```python
from build123d import *

# Parameters (mm, degrees)
EXTRUSION1_REACH = 19.5
ESQUISSE2_R      = 2


with BuildPart() as part:
    # Esquisse1 → Révolution1 (revolve)
    with BuildSketch(Plane.XY):
        Polygon((-17.5, 5), (-4, 5), (-4, 3), (-11, 3), (-11, -21), (-17.5, -21), align=None)
    revolve(axis=Axis((0, 0, 0), (0, -1, 0)))

    # Esquisse2 → Extrusion1 (cut, up to next)
    with BuildSketch(Plane(origin=(0, 0, 0), x_dir=(0, 0, -1), z_dir=(1, 0, 0)), mode=Mode.PRIVATE) as extrusion1_sk1:
        with Locations((0, -13.5)):
            Circle(ESQUISSE2_R)
    extrusion1_tool1 = extrude(extrusion1_sk1.sketch, amount=-EXTRUSION1_REACH, mode=Mode.PRIVATE) & part.part
    add(extrusion1_tool1.solids().sort_by_distance((0, -13.5, 0))[0], mode=Mode.SUBTRACT)


solid = part.part
```
Could you check a few things on this model? Use its own coordinates, in mm. A direction names the side the tool comes from. Round coordinates to 2 decimals unless told otherwise and drop trailing zeros. Write each loop counter-clockwise with the first axis right and the second up, starting at its lowest first coordinate (ties: lowest second). Pieces come first, ordered by that corner, then holes. Notation, with made-up numbers: M 55.5,11.5 L 78.5,11.5 A22 ccw 78.5,36.5 Z; hole C 56,46 d5. An arc over 180 degrees is marked long. Write each question's results on one line, items separated by ' | '. Start each with the question number.
1. Imagine slicing it at B-B on x = 0. List the corners of the cut face in (y, z) for me, and give its area (3 significant figures).
2. Imagine slicing it at D-D on x = 9.5. List the corners of the cut face in (y, z) for me, and give its area (3 significant figures).
3. I'm going to push flat-ended pins straight in: pin 1 Ø5 at (y, z) = (-17.5, 13.5) entering from -X; pin 2 Ø10 at (x, y) = (-6, -14.5) entering from -Z; pin 3 Ø1 at (y, z) = (-0.5, -2.5) entering from +X. Where does each tip first touch, or does it pass through?
4. I need wall thicknesses on L1, parallel to X at y = -5, z = 0; L2, parallel to X at y = 3.9, z = 0. Which ranges of each line are inside material? Lowest first, please. Write a range as from..to.
5. On a 3-axis mill with a long thin cutter (end or side, diameter ignored), from which of +Z, -Z, +X, -X, +Y, -Y can I reach the whole of each face in a straight line? I mean faces 5 (the face through (2.38, -9.17, 10.74)), 6 (the face through (13.887, -7.818, 10.648)). Say none if no direction works.
6. Imagine slicing it at C-C on y = -1.25. List the corners of the cut face in (x, z) for me, and give its area (3 significant figures).
7. Imagine slicing it at A-A on z = 0. List the corners of the cut face in (x, y) for me.
8. Thinking about a two-plate mould opening in Y: for faces 1 (the face through (0.867, 3.986, 3.905)), 2 (the face through (-4, 5, 4)), 3 (the face through (-8, -21, 8)), 4 (the face through (-14.111, -11.517, 0.26)), which applies, +Y half, -Y half, draft (parallel to the pull), parting line (faces both ways), or undercut?
Result sheet:
1) outline: M -21,-17.5 L 5,-17.5 L 5,-4 L 3,-4 L 3,-11 L -21,-11 Z; M -21,11 L 3,11 L 3,4 L 5,4 L 5,17.5 L -21,17.5 Z | area: 366 mm^2
2) outline: M -21,-14.7 L 5,-14.7 L 5,14.7 L -21,14.7 L -21,5.55 L 3,5.55 L 3,-5.55 L -21,-5.55 Z | area: 498 mm^2
3) pin 1: stops at x = -13.61 | pin 2: stops at z = -17.47 | pin 3: stops at x = 17.39
4) L1: x = -17.5..-11, 11..17.5 | L2: x = -17.5..-4, 4..17.5
5) face 5: -Y | face 6: +Y, -Y
6) outline: C 0,0 d35; hole C 0,0 d22 | area: 582 mm^2
7) outline: M -17.5,-21 L -11,-21 L -11,-15.5 L -17.5,-15.5 Z; M -17.5,-11.5 L -11,-11.5 L -11,3 L -4,3 L -4,5 L -17.5,5 Z; M 4,3 L 11,3 L 11,-21 L 17.5,-21 L 17.5,5 L 4,5 Z
8) face 1: draft | face 2: +Y half | face 3: -Y half | face 4: undercut
